Build history of the part. All positions in model axes, mm. A direction names the side the tool comes from. Round coordinates to 2 decimals unless told otherwise and drop trailing zeros. Write each loop counter-clockwise with the first axis right and the second up, starting at its lowest first coordinate (ties: lowest second). Pieces come first, ordered by that corner, then holes.
Item 1: Band-saw the part on B-B, the plane y = 18. Write the cut outline in (x, z), then the cut area to 3 significant figures.
Item 2: Band-saw the part on A-A, the plane x = 0. Write the cut outline in (y, z), then the cut area to 3 significant figures.
Item 3: Band-saw the part on C-C, the plane x = 21.5. Write the cut outline in (y, z).
Item 4: 3-axis set-ups, long thin cutter, end or side, ignore diameter. For faces 5 (the flat face through (11.345, -6.349, 0.493)), 6 (the flat face through (0, 15, 1)): which of +Z, -Z, +X, -X, +Y, -Y reach the whole face in a straight line?
Item 5: Wall check: probe 1 along X at (y, z) = (-9, 0.5); probe 2 along Y at (x, z) = (-16, 0.1); probe 3 along Y at (x, z) = (12.5, 0.75). Give the ranges that are in metal, low to high.
Item 6: Band-saw the part on D-D, the plane z = 0.7. Write the cut outline in (x, y).
Item 7: Mould opens along X. For faces 1 (the cylindrical face through (-15.624, 8.938, 0.493)), 2 (the flat face through (-20.05, -11.27, 0.49)), 3 (the flat face through (0, 15, 0)), 4 (the flat face through (20.05, -11.27, 0.49)) say: +X half, -X half, draft (parallel to the pull), parting line (faces both ways), or undercut.
Autodesk Inventor part; units mm, degrees
ref_plane "YZ Plane" through (0, 0, 0) normal (1, 0, 0) x (0, 1, 0)
ref_plane "XZ Plane" through (0, 0, 0) normal (0, 1, 0) x (-1, 0, 0)
ref_plane "XY Plane" through (0, 0, 0) normal (0, 0, 1) x (1, 0, 0)
sketch "スケッチ1" plane through (0, 0, 0) normal (0, 0, 1) x (1, 0, 0)
  arc A0 (29.5493, 5.1808) -> (19.2614, 23) centre (0, 0) ccw
  arc A1 (-19.2614, 23) -> (-29.5493, 5.1808) centre (0, 0) ccw
  arc A2 (-10.2879, -28.1808) -> (10.2879, -28.1808) centre (0, 0) ccw
  line L0 (29.5493, 5.1808) -> (10.2879, -28.1808)
  line L1 (0, 23) -> (19.2614, 23)
  line L2 (19.9186, -11.5) -> (29.5493, 5.1808)
  line L3 (-19.9186, -11.5) -> (-29.5493, 5.1808)
  line L4 (19.2614, 23) -> (-19.2614, 23)
  line L5 (-29.5493, 5.1808) -> (-10.2879, -28.1808)
  arc A3 (17.4833, 4.2819) -> (12.4499, 13) centre (0, 0) ccw
  arc A4 (-12.4499, 13) -> (-17.4833, 4.2819) centre (0, 0) ccw
  arc A5 (-5.0334, -17.2819) -> (5.0334, -17.2819) centre (0, 0) ccw
  line L6 (0, 13) -> (12.4499, 13)
  line L7 (17.4833, 4.2819) -> (5.0334, -17.2819)
  line L8 (-11.2583, -6.5) -> (-17.4833, 4.2819)
  line L9 (0, 13) -> (-12.4499, 13)
  line L10 (-17.4833, 4.2819) -> (-5.0334, -17.2819)
  point P0 (11.2583, -6.5)
  dimension "d10" = 360
  dimension "d6" = 23
extrude "押し出し1" add sketch "スケッチ1" along normal blind 1
sketch "スケッチ2" plane through (0, 0, 1) normal (0, 0, 1) x (1, 0, 0)
  point P0 (0, 0)
  point P1 (0, 18)
  point P2 (0, 0)
  point P3 (-15.5885, -9)
  point P4 (0, 0)
  point P5 (15.5885, -9)
  point P6 (0, -26)
  point P7 (22.5167, 13)
  point P8 (-22.5167, 13)
  dimension "d15" = 18
  dimension "d18" = 360
  dimension "d20" = 26
  dimension "d23" = 360
hole "穴1" at (0, 18, 1) at (-15.5885, -9, 1) at (15.5885, -9, 1) at (0, -26, 1) at (22.5167, 13, 1) at (-22.5167, 13, 1) direction (0, 0, -1) diameter 3.5 end through all
properties part number "スプリングフランジ"
Results:
1. outline: (-24, 0) - (-1.75, 0) - (-1.75, 1) - (-24, 1) - close; (1.75, 0) - (24, 0) - (24, 1) - (1.75, 1) - close
1. area: 44.5 mm2
2. outline: (-30, 0) - (-27.75, 0) - (-27.75, 1) - (-30, 1) - close; (-24.25, 0) - (-18, 0) - (-18, 1) - (-24.25, 1) - close; (13, 0) - (16.25, 0) - (16.25, 1) - (13, 1) - close; (19.75, 0) - (23, 0) - (23, 1) - (19.75, 1) - close
2. area: 15.0 mm2
3. outline: (-8.76, 0) - (11.58, 0) - (11.58, 1) - (-8.76, 1) - close; (14.42, 0) - (20.92, 0) - (20.92, 1) - (14.42, 1) - close
4. face 5: +Z, -Z
4. face 6: +Z, +X, -X, +Y, -Y
5. probe 1: x = -21.36 to -17.34, -13.84 to -9.81, 9.81 to 13.84, 17.34 to 21.36
5. probe 2: y = -18.29 to -10.7, -7.3 to 1.71, 8.25 to 23
5. probe 3: y = -24.35 to -4.35, 12.95 to 23
6. outline: (-29.55, 5.18) - (-10.29, -28.18) arc R30 ccw to (10.29, -28.18) - (29.55, 5.18) arc R30 ccw to (19.26, 23) - (-19.26, 23) arc R30 ccw to start; hole circle Ø3.5 at (-22.52, 13); hole (-17.48, 4.28) - (-11.26, -6.5) - (-5.03, -17.28) arc R18 ccw to (5.03, -17.28) - (17.48, 4.28) arc R18 ccw to (12.45, 13) - (-12.45, 13) arc R18 ccw to start; hole circle Ø3.5 at (-15.59, -9); hole circle Ø3.5 at (0, -26); hole circle Ø3.5 at (0, 18); hole circle Ø3.5 at (15.59, -9); hole circle Ø3.5 at (22.52, 13)
7. face 1: undercut
7. face 2: -X half
7. face 3: draft
7. face 4: +X half
